```python
from build123d import *

# Parameters (mm, degrees)
SKETCH_R  = 5
PAD_DEPTH = 13


with BuildPart() as part:
    # Sketch → Pad (new body)
    with BuildSketch(Plane.XY):
        Polygon((-13.75, 15), (13.749989, 15), (19.455317, 7.392933), (4.310835, -22), (1.95122, -22), (-1.95122, -22), (-4.310835, -22), (-19.45531, 7.39292), align=None)
        Circle(SKETCH_R, mode=Mode.SUBTRACT)
    pad = extrude(amount=PAD_DEPTH)

    # Mirrored: Pad across Sketch V_Axis
    add(pad.mirror(Plane(origin=(0, 0, 0), x_dir=(0, 0, 1), z_dir=(1, 0, 0))))


solid = part.part
```
Geometry check sheet. Reference: the model listing, model coordinates, mm. Give positions to 0.01 mm unless a question says otherwise; leave off trailing zeros. Loops run counter-clockwise (first coordinate to the right, second up) from the corner with the lowest first, then second, coordinate; pieces in that order, holes last. Notation, with made-up numbers: M -2,72.25 L 16,72.25 A19 ccw 16,82.25 Z; hole C 54.25,14 d11. An arc over 180 degrees is marked long. Write item = value, one per line. Start each with the question number.
1. Section check C-C, the plane y = 0. Enter the section's corners in (x, z), plus the area to 3 significant figures.
2. Section check B-B, the plane z = 1.5. Enter the section's corners in (x, y).
3. Section check A-A, the plane x = 0. Enter the section's corners in (y, z).
4. Go/stop test with flat-tipped pins: P1, Ø5, axis at x = -3, y = 3, coming from the -Z side; P2, Ø2, axis at y = 1, z = 4, coming from the +X side; P3, Ø6, axis at x = -10, z = 11, coming from the -Y side. Record where each tip stops, or that it passes through.
5. Section check D-D, the plane x = 12. Enter the section's corners in (y, z), plus the area to 3 significant figures.
6. Thickness scan on probe 1 along Y at (x, z) = (0, 6.75); probe 2 along X at (y, z) = (1, 0.75); probe 3 along X at (y, z) = (0, 9.5). Record the ranges inside material, lowest first.
7. Draft check along X on faces 1 (the face through (11.99, -7.1, 6.41)), 2 (the face through (-5, -3, 0)), 3 (the face through (-1.08, -4.88, 6.41)). Enter one of: +X half, -X half, draft (parallel to the pull), parting line (faces both ways), or undercut.
Values follow:
q1.outline = M -15.65,0 L -5,0 L -5,13 L -15.65,13 Z; M 5,0 L 15.65,0 L 15.65,13 L 5,13 Z
q1.area = 277 mm^2
q2.outline = M -19.46,7.39 L -4.31,-22 L 4.31,-22 L 19.46,7.39 L 16.01,11.98 L 13.75,15 L -13.75,15 L -16.01,11.98 Z; hole C 0,0 d10
q3.outline = M -22,0 L -5,0 L -5,13 L -22,13 Z; M 5,0 L 15,0 L 15,13 L 5,13 Z
q4.P1 = 0
q4.P2 = 16.68
q4.P3 = -16.78
q5.outline = M -7.08,0 L 15,0 L 15,13 L -7.08,13 Z
q5.area = 287 mm^2
q6.probe_1 = -22 to -5, 5 to 15
q6.probe_2 = -16.16 to -4.9, 4.9 to 16.16
q6.probe_3 = -15.65 to -5, 5 to 15.65
q7.face_1 = +X half
q7.face_2 = draft
q7.face_3 = undercut
